Print and shaded views of the part. All mm, measured from the part's lowest x, y and z. A direction names the side the tool comes from. Round coordinates to 2 decimals unless told otherwise and drop trailing zeros. Loops run counter-clockwise (first coordinate to the right, second up) from the corner with the lowest first, then second, coordinate; pieces in that order, holes last. Notation, with made-up numbers: (-15, -27.75) - (13, -27.75) arc R22 ccw to (13, -9.75) - close; hole circle Ø6 at (18.5, 86). An arc over 180 degrees is marked (long way). Use one line per item in the form item = value. Start each with the question number.
Q1. Drill centre lines: line 1 (Y direction, x = 4.5, z = 13.5); line 2 (Z direction, x = 16.5, y = 10.5); line 3 (X direction, y = 7.5, z = 2.75). Where is each one in solid material? Low to high.
Q2. Mould opens along Y. For the marked faces 4, 5, 6 and 7 say: released by +Y, released by -Y, zero draft, split by the parting line, or undercut.
Q3. 3-axis set-ups, long thin cutter, end or side, ignore diameter. For the marked faces 1, 2 and 3: which of +Z, -Z, +X, -X, +Y, -Y reach the whole face in a straight line?
Q4. Pin check, flat tips, straight feed: pin 1 (10 mm diameter, centred on x = 5.5, y = 12, fed in from +Z); pin 2 (10 mm diameter, centred on x = 9, y = 8.5, fed in from +Z); pin 3 (8 mm diameter, centred on x = 10.5, y = 12.5, fed in from +Z); pin 4 (4 mm diameter, centred on y = 8.5, z = 13, fed in from +X). Stop position of each tip, or through.
Q5. Saw through at D-D (x = 7). Give the cut face in (y, z), then the cut area to 3 significant figures.
Q6. Saw through at C-C (z = 6.75). Give the cut face in (x, y).
Q7. Saw through at A-A (x = 26). Give the cut face in (y, z).
Q8. Saw through at B-B (z = 17.5). Give the cut face in (x, y).
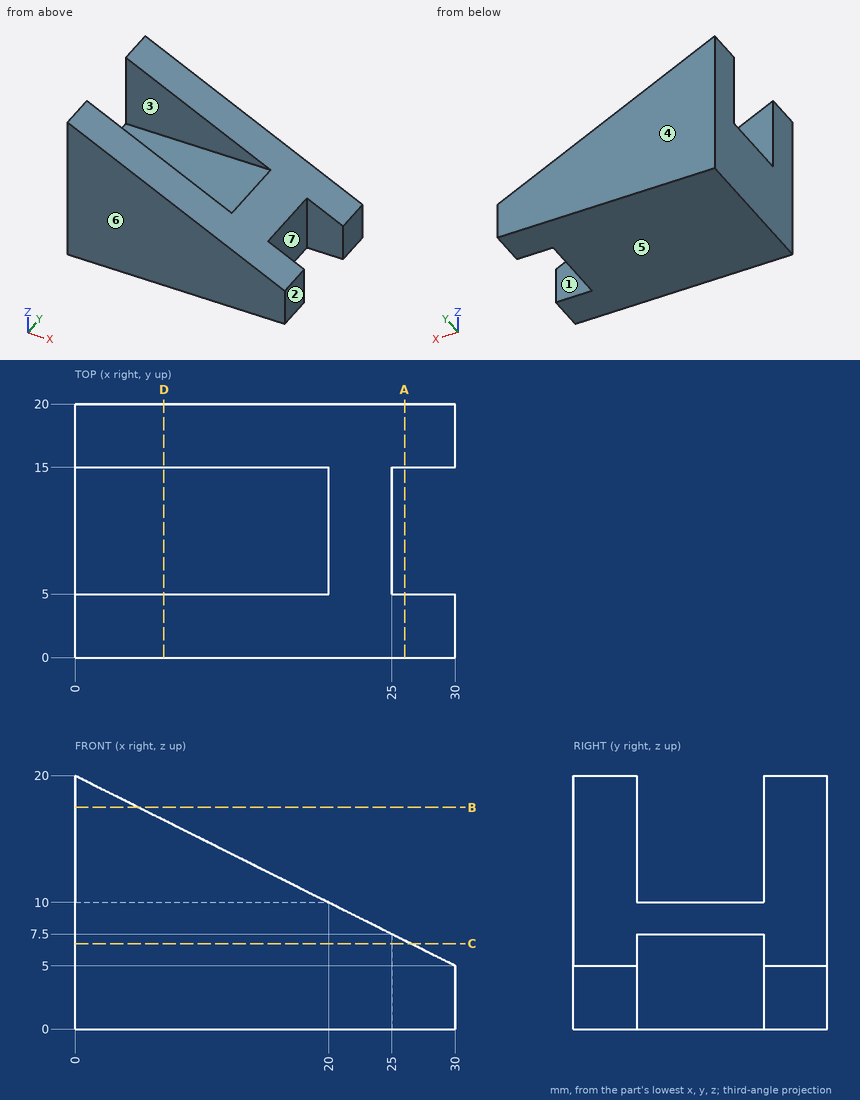
Report:
q1.line_1 = 0 to 5, 15 to 20
q1.line_2 = 0 to 10
q1.line_3 = 0 to 25
q2.face_4 = released by +Y
q2.face_5 = zero draft
q2.face_6 = released by -Y
q2.face_7 = undercut
q3.face_1 = +Z, -Z, +X
q3.face_2 = +Z, -Z, +X, +Y, -Y
q3.face_3 = +Z, +X, -X
q4.pin_1 = 19.25
q4.pin_2 = 17.29
q4.pin_3 = 16.31
q4.pin_4 = through
q5.outline = (0, 0) - (20, 0) - (20, 16.5) - (15, 16.5) - (15, 10) - (5, 10) - (5, 16.5) - (0, 16.5) - close
q5.area = 265 mm²
q6.outline = (0, 0) - (26.5, 0) - (26.5, 5) - (25, 5) - (25, 15) - (26.5, 15) - (26.5, 20) - (0, 20) - close
q7.outline = (0, 0) - (5, 0) - (5, 7) - (0, 7) - close; (15, 0) - (20, 0) - (20, 7) - (15, 7) - close
q8.outline = (0, 0) - (5, 0) - (5, 5) - (0, 5) - close; (0, 15) - (5, 15) - (5, 20) - (0, 20) - close
